Model file for the job. Use its own axes, mm. A direction names the side the tool comes from. Give positions to 0.01 mm unless a question says otherwise; leave off trailing zeros. Write each loop counter-clockwise with the first axis right and the second up, starting at its lowest first coordinate (ties: lowest second). Pieces come first, ordered by that corner, then holes. Notation, with made-up numbers: (20.25, 56) - (75.25, 56) arc R29 cw to (75.25, 85) - close; hole circle Ø6 at (81.25, 85). An arc over 180 degrees is marked (long way). Use a Markdown table: item, result. Add a question column.
```python
from build123d import *

# Parameters (mm, degrees)
SKETCH_1_R          = 5
EXTRUDE_1_DEPTH     = 3
SKETCH_4_R          = 7.5
CUT_EXTRUDE_3_DEPTH = 3


with BuildPart() as part:
    # 草图1 → 凸台-拉伸1 (new body)
    with BuildSketch(Plane.XY):
        with BuildLine():
            Line((0, 12.25), (100, 12.25))
            ThreePointArc((100, 12.25), (112.25, 0), (100, -12.25))
            Line((100, -12.25), (0, -12.25))
            ThreePointArc((0, -12.25), (-12.25, 0), (0, 12.25))
        make_face()
        Circle(SKETCH_1_R, mode=Mode.SUBTRACT)
        with Locations((100, 0)):
            Circle(SKETCH_1_R, mode=Mode.SUBTRACT)
    extrude(amount=EXTRUDE_1_DEPTH)

    # 草图4 → 切除-拉伸3 (cut)
    with BuildSketch(Plane.XY.offset(1)):
        Circle(SKETCH_4_R)
        with Locations((100, 0)):
            Circle(SKETCH_4_R)
    extrude(amount=-CUT_EXTRUDE_3_DEPTH, mode=Mode.SUBTRACT)


solid = part.part
```
(1) Two-plate mould, pull along X, no slides. Class faces 3 (the cylindrical face through (104.619, -1.915, 1.986)), 4 (the flat face through (49, 12.25, 1)), 5 (the cylindrical face through (-12.247, -0.269, 1.479)): +X half, -X half, draft (parallel to the pull), parting line (faces both ways), or undercut.
(2) Band-saw the part on A-A (y = 0). Write the cut outline in (x, z).
(3) Flat gauge pins, fed straight in: pin 1 (1.5 mm diameter, centred on y = -4.5, z = 1.5, fed in from -X); pin 2 (7.5 mm diameter, centred on x = 101.5, y = 1, fed in from -Z). Where does each tip first touch, or does it go through?
(4) Band-saw the part on B-B (z = 2.15). Write the cut outline in (x, y).
(5) Probe probe 1 along X at (y, z) = (0, 2); probe 2 along Y at (x, z) = (100, 2); probe 3 along Y at (x, z) = (100, 0.7). List the from-to ranges inside material, lowest first. Write a range as [from, to].
(6) Band-saw the part on D-D (y = -10.5). Write the cut outline in (x, z), then the cut area to 3 significant figures.
(7) Band-saw the part on C-C (x = 3). Write the cut outline in (y, z), then the cut area to 3 significant figures.
(8) Which spindle directions (+Z, -Z, +X, -X, +Y, -Y) get a long thin tool onto all of the face, cutting with end or side? Do faces 1 (the flat face through (51, 0, 0)), 2 (the cylindrical face through (92.507, 0.33, 0.507)). Say none if no direction does.
Model answer:
| question | item | result |
|---|---|---|
| 1 | face 3 | undercut |
| 1 | face 4 | draft |
| 1 | face 5 | -X half |
| 2 | outline | (-12.25, 0) - (-7.5, 0) - (-7.5, 1) - (-5, 1) - (-5, 3) - (-12.25, 3) - close; (5, 1) - (7.5, 1) - (7.5, 0) - (92.5, 0) - (92.5, 1) - (95, 1) - (95, 3) - (5, 3) - close; (105, 1) - (107.5, 1) - (107.5, 0) - (112.25, 0) - (112.25, 3) - (105, 3) - close |
| 3 | pin 1 | stops at x = -11.66 |
| 3 | pin 2 | stops at z = 1 |
| 4 | outline | (0, -12.25) - (100, -12.25) arc R12.25 ccw to (100, 12.25) - (0, 12.25) arc R12.25 ccw to start; hole circle Ø10 at (0, 0); hole circle Ø10 at (100, 0) |
| 5 | probe 1 | x = [-12.25, -5], [5, 95], [105, 112.25] |
| 5 | probe 2 | y = [-12.25, -5], [5, 12.25] |
| 5 | probe 3 | y = [-12.25, -7.5], [7.5, 12.25] |
| 6 | outline | (-6.31, 0) - (106.31, 0) - (106.31, 3) - (-6.31, 3) - close |
| 6 | area | 338 mm^2 |
| 7 | outline | (-12.25, 0) - (-6.87, 0) - (-6.87, 1) - (-4, 1) - (-4, 3) - (-12.25, 3) - close; (4, 1) - (6.87, 1) - (6.87, 0) - (12.25, 0) - (12.25, 3) - (4, 3) - close |
| 7 | area | 43.8 mm^2 |
| 8 | face 1 | -Z, +X, -X, +Y, -Y |
| 8 | face 2 | -Z |
